Geometry: final body of the model. Coordinates: model frame, mm. Face numbers are marked on the shaded views. A direction names the side the tool comes from. Give positions to 0.01 mm unless a question says otherwise; leave off trailing zeros. Write each loop counter-clockwise with the first axis right and the second up, starting at its lowest first coordinate (ties: lowest second). Pieces come first, ordered by that corner, then holes. Notation, with made-up numbers: (77.25, 56) -> (98.25, 56) arc R7 ccw to (98.25, 66) -> close; hole circle Ø10 at (11.5, 73). An arc over 180 degrees is marked (long way). Answer in a Markdown table with one row per item. Add a question column.
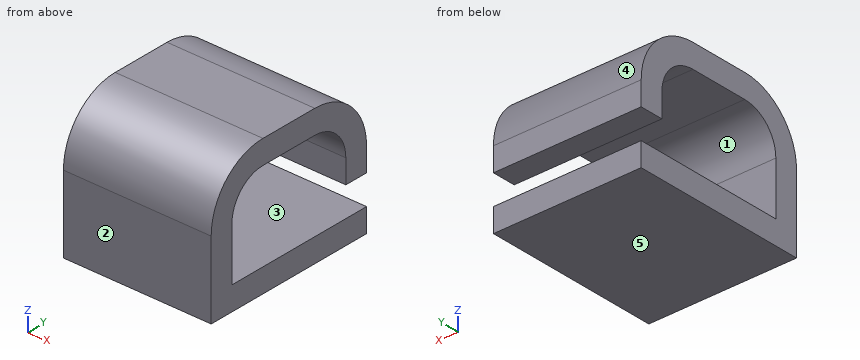
from build123d import *

# Parameters (mm, degrees)
EXTRUDE_1_DEPTH = 5


with BuildPart() as part:
    # Эскиз2 → Бобышка-Вытянуть1 (new body)
    with BuildSketch(Plane(origin=(0, 0, 0), x_dir=(0, 0, -1), z_dir=(1, 0, 0))):
        with BuildLine():
            Line((-3.01866618, 8.509074189), (-3.01866618, 2.509074189))
            Line((-3.01866618, 2.509074189), (-5.61866618, 2.509074189))
            ThreePointArc((-5.61866618, 2.509074189), (-7.032879742, 3.094860626), (-7.61866618, 4.509074189))
            Line((-7.61866618, 4.509074189), (-7.61866618, 6.509074189))
            ThreePointArc((-7.61866618, 6.509074189), (-7.032879742, 7.923287751), (-5.61866618, 8.509074189))
            Line((-5.61866618, 8.509074189), (-4.81866618, 8.509074189))
            Line((-4.81866618, 8.509074189), (-4.81866618, 7.709074189))
            Line((-4.81866618, 7.709074189), (-5.61866618, 7.709074189))
            ThreePointArc((-5.61866618, 7.709074189), (-6.467194317, 7.357602326), (-6.81866618, 6.509074189))
            Line((-6.81866618, 6.509074189), (-6.81866618, 4.509074189))
            ThreePointArc((-6.81866618, 4.509074189), (-6.467194317, 3.660546051), (-5.61866618, 3.309074189))
            Line((-5.61866618, 3.309074189), (-3.81866618, 3.309074189))
            Line((-3.81866618, 3.309074189), (-3.81866618, 8.509074189))
            Line((-3.81866618, 8.509074189), (-3.01866618, 8.509074189))
        make_face()
    extrude(amount=EXTRUDE_1_DEPTH)


solid = part.part
Q1. Section A-A on y = 5.55. Return loops of the section in (x, z), and give its area (3 significant figures).
Q2. Pull-direction query (Z, two-part tool) for the marked faces 3, 4 and 5; classes: +Z half, -Z half, draft (parallel to the pull), parting line (faces both ways), or undercut.
Q3. Access query for the marked faces 1 and 2. Directions: +Z, -Z, +X, -X, +Y, -Y. A direction counts if a zero-diameter tool reaches every point of the face in a straight line with its end or side. Return the directions, or none.
Q4. Section D-D on z = 4.4. Return loops of the section in (x, y), and give its area (3 significant figures).
Q5. Section B-B on z = 5.2. Return loops of the section in (x, y), and give its area (3 significant figures).
Q6. Section C-C on x = 4.65. Return loops of the section in (y, z).
Q7. Line query: probe 1 along Z at (x, y) = (2.3, 6.1); probe 2 along Y at (x, z) = (4.5, 5.55); probe 3 along Y at (x, z) = (2.6, 6.3). Output: solid intervals per line, ascending. Write a range as from..to.
Checks:
| question | item | result |
|---|---|---|
| 1 | outline | (0, 3.02) -> (5, 3.02) -> (5, 3.82) -> (0, 3.82) -> close; (0, 6.82) -> (5, 6.82) -> (5, 7.62) -> (0, 7.62) -> close |
| 1 | area | 8.00 mm^2 |
| 2 | face 3 | undercut |
| 2 | face 4 | +Z half |
| 2 | face 5 | -Z half |
| 3 | face 1 | +X, -X |
| 3 | face 2 | +Z, -Z, +X, -X, -Y |
| 4 | outline | (0, 2.51) -> (5, 2.51) -> (5, 3.31) -> (0, 3.31) -> close |
| 4 | area | 4.00 mm^2 |
| 5 | outline | (0, 2.51) -> (5, 2.51) -> (5, 3.31) -> (0, 3.31) -> close; (0, 7.71) -> (5, 7.71) -> (5, 8.51) -> (0, 8.51) -> close |
| 5 | area | 8.00 mm^2 |
| 6 | outline | (2.51, 3.02) -> (8.51, 3.02) -> (8.51, 3.82) -> (3.31, 3.82) -> (3.31, 5.62) arc R1.2 cw to (4.51, 6.82) -> (6.51, 6.82) arc R1.2 cw to (7.71, 5.62) -> (7.71, 4.82) -> (8.51, 4.82) -> (8.51, 5.62) arc R2 ccw to (6.51, 7.62) -> (4.51, 7.62) arc R2 ccw to (2.51, 5.62) -> close |
| 7 | probe 1 | 3.02..3.82, 6.82..7.62 |
| 7 | probe 2 | 2.51..3.31, 7.71..8.51 |
| 7 | probe 3 | 2.63..3.52, 7.5..8.39 |
